CAD build for the part. Positions are in the model's coordinates, mm. Coordinates: 2 decimals unless noted, no trailing zeros. Write each loop counter-clockwise with the first axis right and the second up, starting at its lowest first coordinate (ties: lowest second). Pieces come first, ordered by that corner, then holes. Notation, with made-up numbers: (31.25, -39.75) -> (76.25, -39.75) arc R26 ccw to (76.25, -23.75) -> close; hole circle Ø8 at (31.25, 40). An arc over 180 degrees is marked (long way). Answer as CSV lines item,"result".
```python
from build123d import *

# Parameters (mm, degrees)
F0_R            = 88.9
F0_R_2          = 14.1605
F1_DEPTH        = 3.175
F2_R            = 2.3622
F3_DEPTH        = 3.176
F3_COPIES_COUNT = 6


# Not quite as in the source:
# - a pattern or mirror of a feature is missing from the dataset's text; its kind, count and spacing are read off the source's solid


with BuildPart() as f1:
    # F0 (on Top) → F1 (new body)
    with BuildSketch(Plane.XY):
        Circle(F0_R)
        Circle(F0_R_2, mode=Mode.SUBTRACT)
    extrude(amount=F1_DEPTH)

    # F2 (on face) → F3 (cut, through all)
    with BuildSketch(Plane.XY.offset(3.175)):
        with Locations((0, 23.8125)):
            Circle(F2_R)
        with Locations((0, 76.2)):
            Circle(F2_R)
        with Locations((25.4, 43.9940905122)):
            Circle(F2_R)
    f3 = extrude(amount=-F3_DEPTH, mode=Mode.SUBTRACT)

    # F3_copies: F3 ×6 about axis
    f3_copies_axis = Axis((0, 0, 0), (0, 0, 1))
    for i in range(1, F3_COPIES_COUNT):
        add(f3.rotate(f3_copies_axis, i * 360 / F3_COPIES_COUNT), mode=Mode.SUBTRACT)


solid = f1.part
```
Item 1: Saw through at B-B on y = -38.1. Give the cut face in (x, z) (3 decimals).
Answer below:
outline,"(-80.322, 0) -> (-68.353, 0) -> (-68.353, 3.175) -> (-80.322, 3.175) -> close; (-63.629, 0) -> (63.629, 0) -> (63.629, 3.175) -> (-63.629, 3.175) -> close; (68.353, 0) -> (80.322, 0) -> (80.322, 3.175) -> (68.353, 3.175) -> close"
Item 2: Saw through at D-D on x = -55.5. Give the cut face in (y, z) (3 decimals), and give its area (3 significant figures).
Answer below:
outline,"(-69.448, 0) -> (69.448, 0) -> (69.448, 3.175) -> (-69.448, 3.175) -> close"
area,"441 mm2"
Item 3: Saw through at A-A on y = -76.2. Give the cut face in (x, z) (1 decimal), and give its area (3 significant figures).
Answer below:
outline,"(-45.8, 0) -> (-2.4, 0) -> (-2.4, 3.2) -> (-45.8, 3.2) -> close; (2.4, 0) -> (45.8, 0) -> (45.8, 3.2) -> (2.4, 3.2) -> close"
area,"276 mm2"
Item 4: Wall check: line 1 (Y direction, x = 0, z = 1.4); line 2 (Y direction, x = -25.4, z = 1.1); line 3 (Y direction, x = -64.5, z = 0.5). Give the ranges that are in metal, low to high. Write a range as from..to.
Answer below:
line 1,"y = -88.9..-78.56, -73.84..-26.17, -21.45..-14.16, 14.16..21.45, 26.17..73.84, 78.56..88.9"
line 2,"y = -85.19..-46.36, -41.63..41.63, 46.36..85.19"
line 3,"y = -61.18..-39.93, -36.27..36.27, 39.93..61.18"
Item 5: Saw through at C-C on z = 2.6. State how many separate pieces and enclosed holes the cut face has, and give its area (3 significant figures).
Answer below:
separate pieces,"1"
enclosed holes,"19"
area,"23,900 mm2"
Item 6: Flat gauge pins, fed straight in: pin 1 (4.5 mm diameter, centred on x = -20.62, y = -11.91, fed in from -Z); pin 2 (1.5 mm diameter, centred on x = -23, z = 0.5, fed in from +Y); pin 3 (1 mm diameter, centred on x = 66, z = 1, fed in from +Y); pin 4 (1.5 mm diameter, centred on y = -62.5, z = 0.5, fed in from +X). Where does each tip first touch, or does it go through?
Answer below:
pin 1,"passes through"
pin 2,"stops at y = 86.07"
pin 3,"stops at y = 60.11"
pin 4,"stops at x = 63.95"
Item 7: Two-plate mould, pull along Y, no slides. Class faces 1 (the cylindrical face through (84.795, 26.703, 1.565)), 2 (the flat face through (19, 1, 0)), 3 (the cylindrical face through (68.35, 38, 1.61)): pulls with the +Y half, pulls with the -Y half, needs draft (parallel to the pull), parting line crosses it, or undercut.
Answer below:
face 1,"parting line crosses it"
face 2,"needs draft"
face 3,"undercut"
